Could you check a few things on this model? Use its own coordinates, in mm. A direction names the side the tool comes from. Coordinates: 2 decimals unless noted, no trailing zeros. Order: outer loops, then holes, each group sorted by start corner. A loop starts at its lowest first (then second) coordinate and runs counter-clockwise, first axis right, second up. Notation, with made-up numbers: (85, 19.25) -> (90, 19.25) arc R18 cw to (90, 29.25) -> close; hole circle Ø4 at (11, 77.5). An arc over 180 degrees is marked (long way). Put each result on its own line as item: value. Start each with the question number.
Q1. Please list where these lines run through material, in increasing order: line 1 along Z through (x, y) = (272, -50) (3 decimals); line 2 along X through (y, z) = (-30.5, 83) (3 decimals); line 3 along Y through (x, z) = (447, 193) (3 decimals).
Q2. Will this pin go through, and if not, where does the flat tip stop? pin 1 (12 mm diameter, centred on x = 85.5, z = 337.5, fed in from -Y) (3 decimals).
Q3. If we section it at C-C (x = 137): Please give me the cut outline in (y, z) (3 decimals).
Q4. If we section it at B-B (z = 359): Please give me the cut outline in (x, y) (3 decimals), and give its area (3 significant figures).
Q5. If we section it at A-A (y = -39): Please give me the cut outline in (x, z) (3 decimals).
Q6. For faces 4 (the face through (257, -42, 406.4)), 5 (the face through (251, -22.225, 206)), which set-ups out of +Z, -Z, +X, -X, +Y, -Y let a thin tool reach every point of the face, with its end or its side?
Q7. We'd pull the mould along Z, two halves only. Please class faces 1 (the face through (257, -52, 384.175)), 2 (the face through (504.38, -42.4, 402.58)), 3 (the face through (504.18, -42.4, 3.62)): +Z half, -Z half, draft (parallel to the pull), parting line (faces both ways), or undercut.
from build123d import *

# Parameters (mm, degrees)
F1_DEPTH = 76.2
F2_T     = -22.225
F3_R     = 9.525
F4_R     = 6.35
F5_R     = 6.35


with BuildPart() as f1:
    # F0 (on Front) → F1 (new body)
    with BuildSketch(Plane.XZ):
        with BuildLine():
            ThreePointArc((0, 12.7), (3.7197438789, 3.7197438789), (12.7, 0))
            Line((12.7, 0), (495.3, 0))
            ThreePointArc((495.3, 0), (504.2802561211, 3.7197438789), (508, 12.7))
            Line((508, 12.7), (508, 393.7))
            ThreePointArc((508, 393.7), (504.2802561211, 402.6802561211), (495.3, 406.4))
            Line((495.3, 406.4), (12.7, 406.4))
            ThreePointArc((12.7, 406.4), (3.7197438789, 402.6802561211), (0, 393.7))
            Line((0, 393.7), (0, 12.7))
        make_face()
    extrude(amount=F1_DEPTH)

    # F2
    f2_openings = [f1.faces().sort_by_distance(p)[0] for p in [
        (254, -76.2, 203.2),
    ]]
    offset(amount=F2_T, openings=f2_openings)

    # F3
    f3_edges = [f1.edges().sort_by_distance(p)[0] for p in [
        (254, 0, 406.4),
    ]]
    fillet(f3_edges, radius=F3_R)

    # F4
    f4_edges = [f1.edges().sort_by_distance(p)[0] for p in [
        (22.225, -49.2125, 22.225),
        (485.775, -49.2125, 22.225),
        (485.775, -49.2125, 384.175),
        (22.225, -49.2125, 384.175),
    ]]
    fillet(f4_edges, radius=F4_R)

    # F5
    f5_edges = [f1.edges().sort_by_distance(p)[0] for p in [
        (22.225, -22.225, 203.2),
    ]]
    fillet(f5_edges, radius=F5_R)


solid = f1.part
The answers:
1. line 1: 0 to 22.225, 384.175 to 406.4
1. line 2: 0 to 22.225, 485.775 to 508
1. line 3: -22.225 to 0
2. pin 1: y = -22.225
3. outline: (-76.2, 0) -> (-9.525, 0) arc R9.525 ccw to (0, 9.525) -> (0, 396.875) arc R9.525 ccw to (-9.525, 406.4) -> (-76.2, 406.4) -> (-76.2, 384.175) -> (-28.575, 384.175) arc R6.35 cw to (-22.225, 377.825) -> (-22.225, 28.575) arc R6.35 cw to (-28.575, 22.225) -> (-76.2, 22.225) -> close
4. outline: (0, -76.2) -> (22.225, -76.2) -> (22.225, -28.575) arc R6.35 cw to (28.575, -22.225) -> (479.425, -22.225) arc R6.35 cw to (485.775, -28.575) -> (485.775, -76.2) -> (508, -76.2) -> (508, -9.525) arc R9.525 ccw to (498.475, 0) -> (9.525, 0) arc R9.525 ccw to (0, -9.525) -> close
4. area: 13,700 mm^2
5. outline: (0, 12.7) arc R12.7 ccw to (12.7, 0) -> (495.3, 0) arc R12.7 ccw to (508, 12.7) -> (508, 393.7) arc R12.7 ccw to (495.3, 406.4) -> (12.7, 406.4) arc R12.7 ccw to (0, 393.7) -> close; hole (22.225, 28.575) arc R6.35 ccw to (28.575, 22.225) -> (479.425, 22.225) arc R6.35 ccw to (485.775, 28.575) -> (485.775, 377.825) arc R6.35 ccw to (479.425, 384.175) -> (28.575, 384.175) arc R6.35 ccw to (22.225, 377.825) -> close
6. face 4: +Z, +X, -X, +Y, -Y
6. face 5: -Y
7. face 1: undercut
7. face 2: +Z half
7. face 3: -Z half
